Build history of the part. All positions in model axes, mm. A direction names the side the tool comes from. Coordinates: 2 decimals unless noted, no trailing zeros. Write each loop counter-clockwise with the first axis right and the second up, starting at its lowest first coordinate (ties: lowest second). Pieces come first, ordered by that corner, then holes.
from build123d import *

# Parameters (mm, degrees)
ESQUISSE1_W              = 60
ESQUISSE1_H              = 6
BOSS_EXTRU_1_DEPTH       = 60
ESQUISSE2_R              = 1.25
ENL_V_MAT_EXTRU_1_DEPTH  = 10
ESQUISSE3_R              = 1.25
ENL_V_MAT_EXTRU_2_DEPTH  = 15
ESQUISSE4_W              = 10
ESQUISSE4_H              = 11
ENL_V_MAT_EXTRU_3_DEPTH  = 3
ENL_V_MAT_EXTRU_4_DEPTH  = 52
CHANFREIN1_SIZE2         = 6.433520762
CHANFREIN1_SIZE          = 3
ESQUISSE6_W              = 2
ESQUISSE6_H              = 5
ENL_V_MAT_EXTRU_16_DEPTH = 2.99


with BuildPart() as part:
    # Esquisse1 → Boss.-Extru.1 (new body)
    with BuildSketch(Plane.XY):
        with Locations((30, 3)):
            Rectangle(ESQUISSE1_W, ESQUISSE1_H)
    extrude(amount=BOSS_EXTRU_1_DEPTH)

    # Esquisse2 → Enlèv. mat.-Extru.1 (cut)
    with BuildSketch(Plane(origin=(0, 0, 0), x_dir=(-1, 0, 0), z_dir=(0, 0, -1))):
        with Locations((-54, 3)):
            Circle(ESQUISSE2_R)
        with Locations((-5.75, 3)):
            Circle(ESQUISSE2_R)
    extrude(amount=-ENL_V_MAT_EXTRU_1_DEPTH, mode=Mode.SUBTRACT)

    # Esquisse3 → Enlèv. mat.-Extru.2 (cut)
    with BuildSketch(Plane(origin=(0, 6, 0), x_dir=(1, 0, 0), z_dir=(0, 1, 0))):
        with Locations(Location((28.75, -37.5, 0), (0, 0, 270))):
            Circle(ESQUISSE3_R)
    extrude(amount=-ENL_V_MAT_EXTRU_2_DEPTH, mode=Mode.SUBTRACT)

    # Esquisse4 → Enlèv. mat.-Extru.3 (cut)
    with BuildSketch(Plane(origin=(0, 6, 0), x_dir=(1, 0, 0), z_dir=(0, 1, 0))):
        Polygon((0, -16), (9, -16), (9, 0), (51, 0), (51, -16), (60, -16), (60, -60), (0, -60), align=None)
        with Locations((28.75, -37.5)):
            Rectangle(ESQUISSE4_W, ESQUISSE4_H, mode=Mode.SUBTRACT)
    extrude(amount=-ENL_V_MAT_EXTRU_3_DEPTH, mode=Mode.SUBTRACT)

    # Esquisse5 → Enlèv. mat.-Extru.4 (cut)
    with BuildSketch(Plane(origin=(0, 3, 0), x_dir=(1, 0, 0), z_dir=(0, 1, 0))):
        Polygon((60, -16), (33.75, -32), (33.75, -43), (23.75, -43), (23.75, -32), (0, -16), (-21.594855386, -85.475485762), (75.414479662, -69.930764824), align=None)
    extrude(amount=-ENL_V_MAT_EXTRU_4_DEPTH, mode=Mode.SUBTRACT)

    # Chanfrein1
    chanfrein1_edges = [part.edges().sort_by_distance(p)[0] for p in [
        (28.75, 3, 32),
    ]]
    chanfrein1_side = [part.faces().sort_by_distance(p)[0] for p in [
        (28.75, 3.06, 32),
    ]]
    chamfer(chanfrein1_edges, length=CHANFREIN1_SIZE - 0.0001, length2=CHANFREIN1_SIZE2 - 0.0001, reference=chanfrein1_side[0])  # a hair under: the kernel refuses the full size

    # Esquisse6 → Enlèv. mat.-Extru.16 (cut)
    with BuildSketch(Plane(origin=(0, 6, 0), x_dir=(1, 0, 0), z_dir=(0, 1, 0))):
        with Locations((52, -13.5)):
            Rectangle(ESQUISSE6_W, ESQUISSE6_H)
        with Locations((8, -13.5)):
            Rectangle(ESQUISSE6_W, ESQUISSE6_H)
    extrude(amount=-ENL_V_MAT_EXTRU_16_DEPTH, mode=Mode.SUBTRACT)


solid = part.part
(1) Slice it at A-A, the plane z = 37.5. List the corners of the cut face in (x, y), and give its area (3 significant figures).
(2) Slice it at B-B, the plane y = 5.35. List the corners of the cut face in (x, z).
(3) 3-axis set-ups, long thin cutter, end or side, ignore diameter. For faces 4 (the flat face through (33.75, 3, 37)), 5 (the flat face through (6, 3, 10)), 6 (the flat face through (8, 5, 11)), 7 (the flat face through (30, 2, 0)): which of +Z, -Z, +X, -X, +Y, -Y reach the whole face in a straight line?
(4) Flat gauge pins, fed straight in: P1, Ø1, axis at x = 8, z = 13.5, coming from the +Y side; P2, Ø2.5, axis at x = 53.5, y = 4.5, coming from the +Z side; P3, Ø1.8, axis at y = 3, z = 36.5, coming from the -X side. Where does each tip first touch, or does it go through?
(5) Probe L1, parallel to X at y = 5.5, z = 7; L2, parallel to X at y = 3.45, z = 12; L3, parallel to Y at x = 5.75, z = 4.25. List the from-to ranges inside material, lowest first.
(6) Slice it at D-D, the plane z = 9. List the corners of the cut face in (x, y), and give its area (3 significant figures).
(7) Two-plate mould, pull along Y, no slides. Class faces 1 (the cylindrical face through (52.81, 3.38, 4.93)), 2 (the cylindrical face through (28.8, 3.04, 36.25)), 3 (the flat face through (30, 0, 16)): pulls with the +Y half, pulls with the -Y half, needs draft (parallel to the pull), parting line crosses it, or undercut.
Results:
1. outline: (23.75, 0) - (27.5, 0) - (27.5, 6) - (23.75, 6) - close; (30, 0) - (33.75, 0) - (33.75, 6) - (30, 6) - close
1. area: 45.0 mm2
2. outline: (0, 0) - (9, 0) - (9, 11) - (7, 11) - (7, 16) - (0, 16) - close; (21.68, 30.61) - (36.04, 30.61) - (33.75, 32) - (33.75, 43) - (23.75, 43) - (23.75, 32) - close; (51, 0) - (60, 0) - (60, 16) - (53, 16) - (53, 11) - (51, 11) - close; hole circle Ø2.5 at (28.75, 37.5)
3. face 4: +Z, +X, +Y, -Y
3. face 5: -Z
3. face 6: +Z, +Y
3. face 7: -Z, +X, -X, +Y, -Y
4. P1: stops at y = 3.01
4. P2: stops at z = 16
4. P3: stops at x = 23.75
5. L1: x = 0 to 9, 51 to 60
5. L2: x = 0 to 7, 53 to 60
5. L3: y = 0 to 1.75, 4.25 to 6
6. outline: (0, 0) - (60, 0) - (60, 6) - (51, 6) - (51, 3) - (9, 3) - (9, 6) - (0, 6) - close; hole circle Ø2.5 at (5.75, 3); hole circle Ø2.5 at (54, 3)
6. area: 224 mm2
7. face 1: undercut
7. face 2: needs draft
7. face 3: pulls with the -Y half
